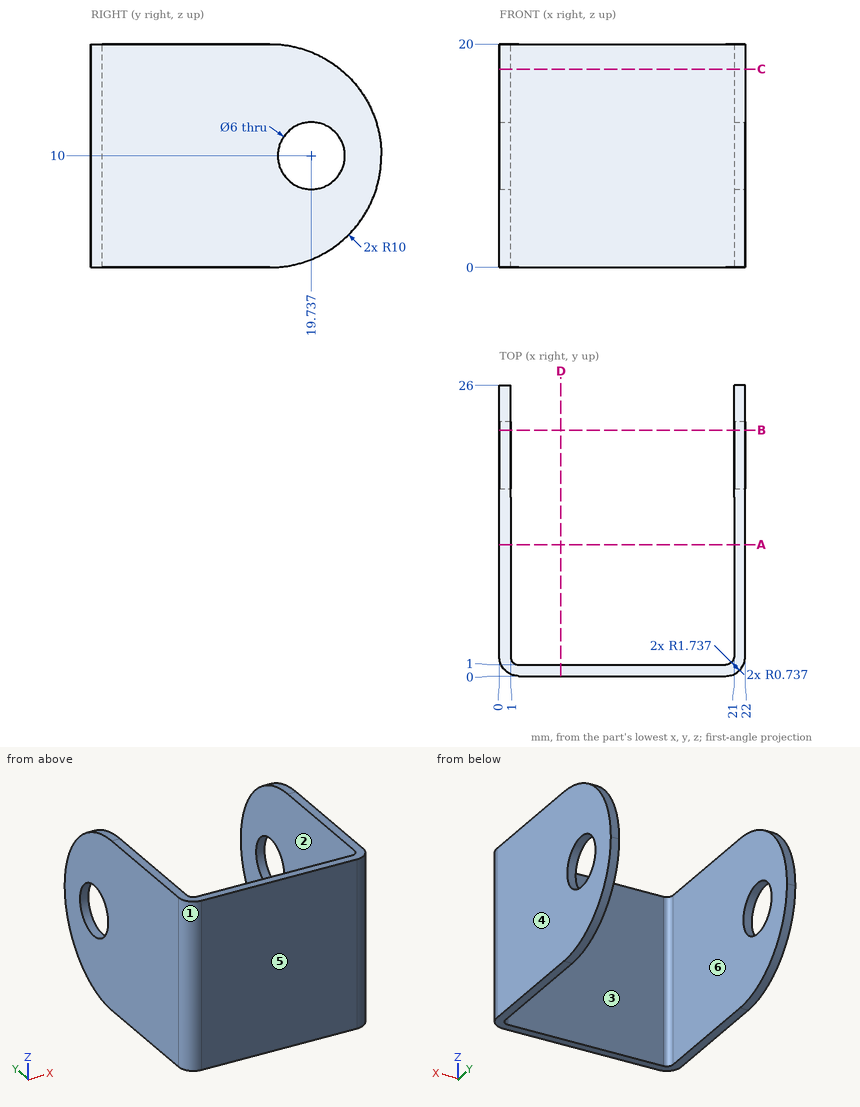
Design review of the part shown in the three views and the two pictorial views. Dimensions are in mm from the part's minimum x, y and z. A direction names the side the tool comes from. Round coordinates to 2 decimals unless told otherwise and drop trailing zeros. Loops run counter-clockwise (first coordinate to the right, second up) from the corner with the lowest first, then second, coordinate; pieces in that order, holes last. Notation, with made-up numbers: (-13, 26.5) - (43, 26.5) arc R13 ccw to (43, 39.5) - close; hole circle Ø1 at (74, 84). An arc over 180 degrees is marked (long way). Use CSV: the item, a comma, the result in double quotes.
(1) Take a section at A-A, the plane y = 11.75. Give the boundary of the cut face in (x, z).
Working result:
outline,"(0, 0) - (1, 0) - (1, 20) - (0, 20) - close; (21, 0) - (22, 0) - (22, 20) - (21, 20) - close"
(2) Take a section at D-D, the plane x = 5.5. Give the boundary of the cut face in (y, z), plus the area to 3 significant figures.
Working result:
outline,"(0, 0) - (1, 0) - (1, 20) - (0, 20) - close"
area,"20.0 mm^2"
(3) Clearance check with flat-ended pins moving along their axes: P1, Ø1.5, axis at x = 2.5, z = 6, coming from the +Y side; P2, Ø5, axis at x = 4.5, y = 21.5, coming from the -Z side. State where each tip first meets the part, or that it passes through.
Working result:
P1,"stops at y = 1"
P2,"passes through"
(4) For line 1 (X direction, y = 20, z = 17.5); line 2 (Y direction, x = 8, z = 9.75), list the stretches that pass through material, from the lowest coordinate up.
Working result:
line 1,"x = 0 to 1, 21 to 22"
line 2,"y = 0 to 1"
(5) Take a section at C-C, the plane z = 17.75. Give the boundary of the cut face in (x, y).
Working result:
outline,"(0, 1.74) arc R1.74 ccw to (1.74, 0) - (20.26, 0) arc R1.74 ccw to (22, 1.74) - (22, 22.32) - (21, 22.32) - (21, 1.74) arc R0.74 cw to (20.26, 1) - (1.74, 1) arc R0.74 cw to (1, 1.74) - (1, 22.32) - (0, 22.32) - close"
(6) Take a section at B-B, the plane y = 22. Give the boundary of the cut face in (x, z).
Working result:
outline,"(0, 2) - (1, 2) - (1, 8.03) - (0, 8.03) - close; (0, 11.97) - (1, 11.97) - (1, 18) - (0, 18) - close; (21, 2) - (22, 2) - (22, 8.03) - (21, 8.03) - close; (21, 11.97) - (22, 11.97) - (22, 18) - (21, 18) - close"
(7) Machinability: for the marked faces 5 and 6, which of the approach directions +Z, -Z, +X, -X, +Y, -Y give a long, thin tool a straight path to every point of the face, cutting with its end or side? Answer none if there is none.
Working result:
face 5,"+Z, -Z, +X, -X, -Y"
face 6,"+Z, -Z, +Y"
(8) The part is to be moulded in two halves that separate along X. For the marked faces 1, 2, 3 and 4, say which applies: pulls with the +X half, pulls with the -X half, needs draft (parallel to the pull), parting line crosses it, or undercut.
Working result:
face 1,"pulls with the -X half"
face 2,"undercut"
face 3,"undercut"
face 4,"pulls with the +X half"
